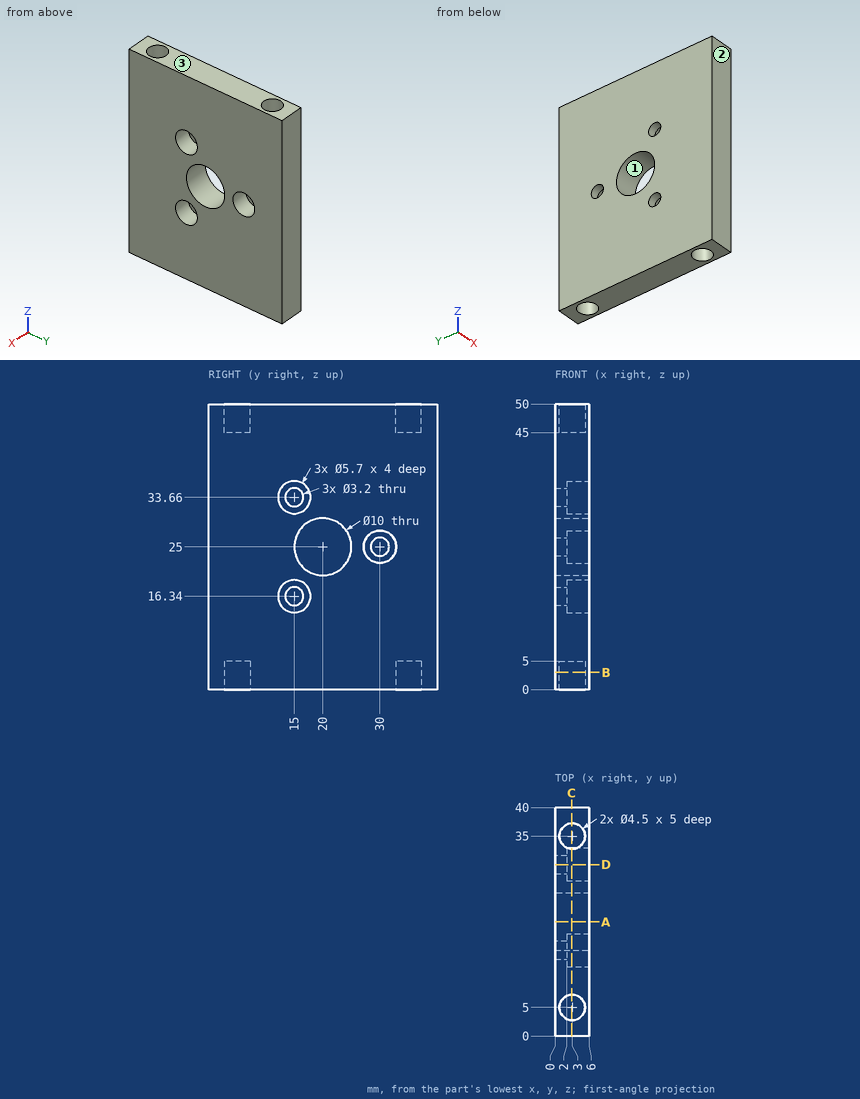
Study the drawing (mm; zero at the part's minimum x, y, z) and answer. Give positions to 0.01 mm unless a question says otherwise; leave off trailing zeros. Write each loop counter-clockwise with the first axis right and the second up, starting at its lowest first coordinate (ties: lowest second). Pieces come first, ordered by that corner, then holes. Notation, with made-up numbers: (26.5, 22.5) -> (30.5, 22.5) arc R33 ccw to (30.5, 61.5) -> close; hole circle Ø5 at (64, 51.25). An arc over 180 degrees is marked (long way). Answer as a JSON object with one key per item and string values. Group by question number.
1) Find section A-A (y = 20). Write down the section's boundary in (x, z), and give its area (3 significant figures).
2) Find section D-D (y = 30). Write down the section's boundary in (x, z).
3) Consider L1, parallel to Y at x = 3, z = 1.95; L2, parallel to Z at x = 2.75, y = 16; L3, parallel to Z at x = 2.7, y = 14. Determine where each line is inside the solid, lowest interval first. Write a range as from..to.
4) Find section B-B (z = 3). Write down the section's boundary in (x, y), and give its area (3 significant figures).
5) The mould has two halves that part along Y. Classify the marked faces 1, 2 and 3: +Y half, -Y half, draft (parallel to the pull), parting line (faces both ways), or undercut.
6) Find section C-C (x = 2.9). Write down the section's boundary in (y, z), and give its area (4 significant figures).
7) Each of these flat-tipped pins is pushed along its axis until it touches: P1, Ø2, axis at x = 2, z = 40, coming from the -Y side; P2, Ø1.7, axis at y = 31, z = 25.5, coming from the +X side; P3, Ø1.3, axis at x = 4, y = 4.5, coming from the -Z side. Where does it stop, or does it pass through?
Values follow:
{
 "1": {"outline": "(0, 0) -> (6, 0) -> (6, 20) -> (0, 20) -> close; (0, 30) -> (6, 30) -> (6, 50) -> (0, 50) -> close", "area": "240 mm2"},
 "2": {"outline": "(0, 0) -> (6, 0) -> (6, 22.15) -> (2, 22.15) -> (2, 23.4) -> (0, 23.4) -> close; (0, 26.6) -> (2, 26.6) -> (2, 27.85) -> (6, 27.85) -> (6, 50) -> (0, 50) -> close"},
 "3": {"L1": "y = 0..2.75, 7.25..32.75, 37.25..40", "L2": "z = 0..13.67, 19.01..22, 28..30.99, 36.33..50", "L3": "z = 0..13.67, 19.01..30.99, 36.33..50"},
 "4": {"outline": "(0, 0) -> (6, 0) -> (6, 40) -> (0, 40) -> close; hole circle Ø4.5 at (3, 5); hole circle Ø4.5 at (3, 35)", "area": "208 mm2"},
 "5": {"face 1": "undercut", "face 2": "-Y half", "face 3": "draft"},
 "6": {"outline": "(0, 0) -> (2.75, 0) -> (2.75, 5) -> (7.25, 5) -> (7.25, 0) -> (32.75, 0) -> (32.75, 5) -> (37.25, 5) -> (37.25, 0) -> (40, 0) -> (40, 50) -> (37.25, 50) -> (37.25, 45) -> (32.75, 45) -> (32.75, 50) -> (7.25, 50) -> (7.25, 45) -> (2.75, 45) -> (2.75, 50) -> (0, 50) -> close; hole circle Ø5.7 at (15, 16.34); hole circle Ø5.7 at (15, 33.66); hole circle Ø10 at (20, 25); hole circle Ø5.7 at (30, 25)", "area": "1,755 mm2"},
 "7": {"P1": "stops at y = 0", "P2": "stops at x = 2", "P3": "stops at z = 5"}
}
